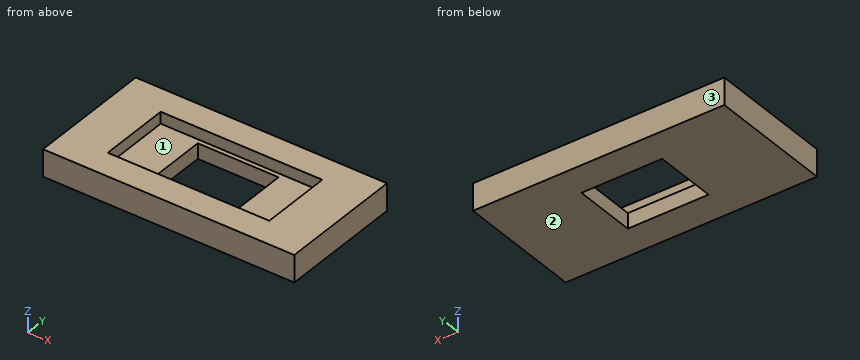
from build123d import *

# Parameters (mm, degrees)
F0_W     = 177.8
F0_H     = 88.9
F1_DEPTH = 19.05
F2_W     = 114.3
F2_H     = 50.8
F3_DEPTH = 8.255
F4_W     = 57.15
F4_H     = 44.45
F5_DEPTH = 19.051


with BuildPart() as f1:
    # F0 (on Top) → F1 (new body)
    with BuildSketch(Plane.XY):
        Rectangle(F0_W, F0_H)
    extrude(amount=F1_DEPTH)

    # F2 (on face) → F3 (cut)
    with BuildSketch(Plane.XY.offset(19.05)):
        Rectangle(F2_W, F2_H)
    extrude(amount=-F3_DEPTH, mode=Mode.SUBTRACT)

    # F4 (on face) → F5 (cut, through all)
    with BuildSketch(Plane(origin=(0, 0, 0), x_dir=(1, 0, 0), z_dir=(0, 0, -1))):
        Rectangle(F4_W, F4_H)
    extrude(amount=-F5_DEPTH, mode=Mode.SUBTRACT)


solid = f1.part
Design review of the part built by this model. Coordinates are the model's own, in mm. Face numbers are marked on the shaded views. Round coordinates to 2 decimals unless told otherwise and drop trailing zeros. Loops run counter-clockwise (first coordinate to the right, second up) from the corner with the lowest first, then second, coordinate; pieces in that order, holes last. Notation, with made-up numbers: (20.25, -1) -> (68.25, -1) arc R25 cw to (68.25, 21) -> close; hole circle Ø11 at (-26, 19.25). An arc over 180 degrees is marked (long way). Use one line per item in the form item = value. Start each with the question number.
Q1. Wall thickness on line 1 along X through (y, z) = (6.5, 10.75) (3 decimals); line 2 along X through (y, z) = (21.5, 13.5); line 3 along Y through (x, z) = (28, 4.25) (3 decimals): over which ranges is each line inside the solid? List them lowest first. Write a range as [from, to].
Q2. Draft analysis for pull direction Y (two halves, no side actions). For the marked faces 1, 2 and 3, state which applies: +Y half, -Y half, draft (parallel to the pull), parting line (faces both ways), or undercut.
Q3. We need section A-A on x = -19. Give the boundary of the cut face in (y, z) (3 decimals), then the cut area to 3 significant figures.
Q4. We need section C-C on y = 4. Give the boundary of the cut face in (x, z) (3 decimals), then the cut area to 3 significant figures.
Q5. We need section B-B on z = 15. Give the boundary of the cut face in (x, y), then the cut area to 4 significant figures.
Q6. We need section D-D on x = 53. Give the boundary of the cut face in (y, z) (3 decimals), then the cut area to 3 significant figures.
Calculated:
q1.line_1 = [-88.9, -28.575], [28.575, 88.9]
q1.line_2 = [-88.9, -57.15], [57.15, 88.9]
q1.line_3 = [-44.45, -22.225], [22.225, 44.45]
q2.face_1 = undercut
q2.face_2 = draft
q2.face_3 = +Y half
q3.outline = (-44.45, 0) -> (-22.225, 0) -> (-22.225, 10.795) -> (-25.4, 10.795) -> (-25.4, 19.05) -> (-44.45, 19.05) -> close; (22.225, 0) -> (44.45, 0) -> (44.45, 19.05) -> (25.4, 19.05) -> (25.4, 10.795) -> (22.225, 10.795) -> close
q3.area = 794 mm²
q4.outline = (-88.9, 0) -> (-28.575, 0) -> (-28.575, 10.795) -> (-57.15, 10.795) -> (-57.15, 19.05) -> (-88.9, 19.05) -> close; (28.575, 0) -> (88.9, 0) -> (88.9, 19.05) -> (57.15, 19.05) -> (57.15, 10.795) -> (28.575, 10.795) -> close
q4.area = 1,830 mm²
q5.outline = (-88.9, -44.45) -> (88.9, -44.45) -> (88.9, 44.45) -> (-88.9, 44.45) -> close; hole (-57.15, -25.4) -> (57.15, -25.4) -> (57.15, 25.4) -> (-57.15, 25.4) -> close
q5.area = 10,000 mm²
q6.outline = (-44.45, 0) -> (44.45, 0) -> (44.45, 19.05) -> (25.4, 19.05) -> (25.4, 10.795) -> (-25.4, 10.795) -> (-25.4, 19.05) -> (-44.45, 19.05) -> close
q6.area = 1,270 mm²
